from build123d import *

# Parameters (mm, degrees)
SKETCH1_R                      = 30.48
BOSS_EXTRUDE1_DEPTH            = 6.35
F_9_0_196_DIAMETER_HOLE1_D     = 4.9784
F_5_16_0_3125_DIAMETER_HOLE1_D = 7.9375


with BuildPart() as part:
    # Sketch1 → Boss-Extrude1 (new body)
    with BuildSketch(Plane(origin=(0, 0, 0), x_dir=(0, 1, 0), z_dir=(0, 0, 1))):
        with BuildLine():
            Line((-59.055, 0), (-59.055, -120.65))
            Line((-59.055, -120.65), (59.055, -120.65))
            Line((59.055, -120.65), (59.055, 0))
            ThreePointArc((59.055, 0), (0, 59.055), (-59.055, 0))
        make_face()
        with Locations(Location((0, 0, 0), (0, 0, 270))):
            Circle(SKETCH1_R, mode=Mode.SUBTRACT)
    extrude(amount=BOSS_EXTRUDE1_DEPTH)

    # #9 (0.196) Diameter Hole1 (through all)
    with Locations(Plane.XY.offset(6.35)):
        with Locations((114.3, -50.8), (101.6, -50.8), (101.6, -38.1), (101.6, -25.4), (101.6, -12.7), (101.6, 0), (101.6, 12.7), (101.6, 25.4), (101.6, 38.1), (101.6, 50.8), (114.3, -38.1), (114.3, -25.4), (114.3, -12.7), (114.3, 0), (114.3, 12.7), (114.3, 25.4), (114.3, 38.1), (114.3, 50.8)):
            Hole(F_9_0_196_DIAMETER_HOLE1_D / 2)

    # 5/16 (0.3125) Diameter Hole1 (through all)
    with Locations(Plane.XY.offset(6.35)):
        with Locations((37.394976935, 21.59), (37.394976935, -21.59), (0, -43.18), (-37.394976935, -21.59), (-37.394976935, 21.59), (0, 43.18)):
            Hole(F_5_16_0_3125_DIAMETER_HOLE1_D / 2)


solid = part.part
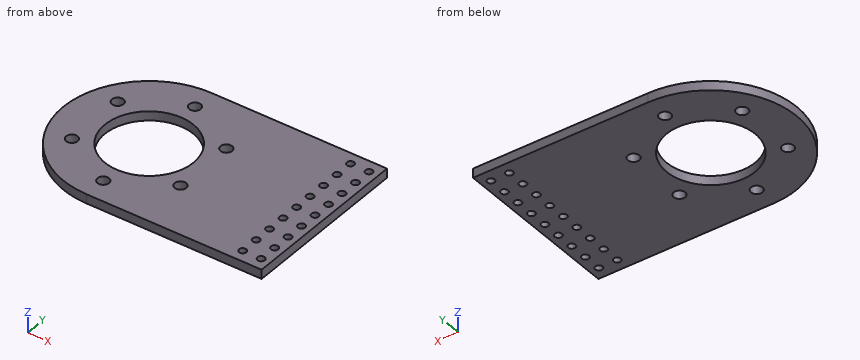
Geometry check sheet. Reference: the model listing, model coordinates, mm. Give positions to 0.01 mm unless a question says otherwise; leave off trailing zeros. Order: outer loops, then holes, each group sorted by start corner. A loop starts at its lowest first (then second) coordinate and runs counter-clockwise, first axis right, second up.
1) Cross-section at C-C (x = 7.5). Record the boundary of the cut face in (y, z) (3 decimals).
Results are:
outline: (-59.055, 0) - (-29.543, 0) - (-29.543, 6.35) - (-59.055, 6.35) - close; (29.543, 0) - (59.055, 0) - (59.055, 6.35) - (29.543, 6.35) - close
2) Cross-section at D-D (y = 50.8). Record the boundary of the cut face in (x, z), then the cut area to 3 significant figures.
Results are:
outline: (-30.11, 0) - (99.11, 0) - (99.11, 6.35) - (-30.11, 6.35) - close; (104.09, 0) - (111.81, 0) - (111.81, 6.35) - (104.09, 6.35) - close; (116.79, 0) - (120.65, 0) - (120.65, 6.35) - (116.79, 6.35) - close
area: 894 mm2
3) Cross-section at B-B (y = -43.18). Record the boundary of the cut face in (x, z).
Results are:
outline: (-40.29, 0) - (-3.97, 0) - (-3.97, 6.35) - (-40.29, 6.35) - close; (3.97, 0) - (120.65, 0) - (120.65, 6.35) - (3.97, 6.35) - close
4) Cross-section at A-A (z = 1.75). Give the number of separate pieces and of enclosed holes in the cut face, then the cut area to 3 significant figures.
Results are:
separate pieces: 1
enclosed holes: 25
area: 16,200 mm2
5) Material ranges on probe 1 along Y at (x, z) = (0, 3.25) (3 decimals); probe 2 along X at (y, z) = (11.5, 1); probe 3 along X at (y, z) = (22.5, 6), recorded low to high.
Results are:
probe 1: y = -59.055 to -47.149, -39.211 to -30.48, 30.48 to 39.211, 47.149 to 59.055
probe 2: x = -57.92 to -28.23, 28.23 to 99.42, 103.78 to 112.12, 116.48 to 120.65
probe 3: x = -54.6 to -41.26, -33.53 to -20.56, 20.56 to 33.53, 41.26 to 120.65
6) Gauge pin test, flat ends, axial feed: pin 1 (2 mm diameter, centred on x = -35, z = 4, fed in from +Y); pin 2 (2 mm diameter, centred on x = -11.5, z = 2.5, fed in from +Y). Record the tip position at first contact, or that the pin passes through.
Results are:
pin 1: stops at y = 48.29
pin 2: stops at y = 58.11
